Verification items for the finished model (mm, model axes). Face numbers are marked on the shaded views. A direction names the side the tool comes from. Give positions to 0.01 mm unless a question says otherwise; leave off trailing zeros. Loops run counter-clockwise (first coordinate to the right, second up) from the corner with the lowest first, then second, coordinate; pieces in that order, holes last. Notation, with made-up numbers: (-26.75, -14) - (29.25, -14) arc R5 ccw to (29.25, -6) - close; hole circle Ø11 at (-11.5, 60). An arc over 180 degrees is marked (long way). One line per item, written item: value. Start each with the question number.
1. Sectioned sample at B-B (z = -12). Record the cut outline in (x, y), plus the area to 3 significant figures.
2. Sectioned sample at A-A (y = 22). Record the cut outline in (x, z), plus the area to 3 significant figures.
3. Mould release check, pull along Y, two halves, no side actions. Record for the marked faces 4, 5, 6 and 7: pulls with the +Y half, pulls with the -Y half, needs draft (parallel to the pull), parting line crosses it, or undercut.
4. Access from +Z, -Z, +X, -X, +Y, -Y to the whole of each face (thin tool, end or side, straight path). Record for the marked faces 1, 2 and 3.
5. Sectioned sample at D-D (y = 45.5). Record the cut outline in (x, z), plus the area to 3 significant figures.
6. Gauge pin test, flat ends, axial feed: pin 1 (7 mm diameter, centred on y = 31, z = -133.5, fed in from +X); pin 2 (7 mm diameter, centred on y = 31, z = -37.5, fed in from -X); pin 3 (7 mm diameter, centred on x = 31.5, z = -161, fed in from +Y); pin 4 (14 mm diameter, centred on x = 16, y = 51, fed in from +Z). Record the tip position at first contact, or that the pin passes through.
7. Scan lines: L1, parallel to Z at x = 11.5, y = 12.75; L2, parallel to X at y = 9.5, z = -162; L3, parallel to Z at x = 13.5, y = 55. Record each from-to range of solid material in increasing order. Write a range as [from, to].
Autodesk Inventor part; units mm, degrees
ref_plane "Work Plane1" through (23, 0, 0) normal (1, 0, 0) x (0, 1, 0)
ref_plane "Work Plane2" through (0, 0, -87) normal (0, 0, 1) x (1, 0, 0)
ref_plane "XZ Plane" through (0, 0, 0) normal (0, 1, 0) x (-1, 0, 0)
sketch "Sketch1" plane through (0, 0, 0) normal (0, 1, 0) x (-1, 0, 0)
  line L0 (0, 0) -> (-46, 0)
  line L1 (-46, 0) -> (-46, -174)
  line L2 (-46, -174) -> (0, -174)
  line L3 (0, -174) -> (0, 0)
  dimension "d0" = 46
  dimension "d1" = 174
extrude "Extrusion1" add sketch "Sketch1" along normal blind 18
sketch "Sketch2" plane through (0, 18, 0) normal (0, 1, 0) x (1, 0, 0)
  line L0 (0, 0) -> (0, 24)
  line L1 (0, 174) -> (0, 0)
  line L2 (46, 0) -> (46, 174)
  line L3 (0, 24) -> (46, 24)
  line L4 (46, 24) -> (46, 55)
  line L5 (46, 55) -> (0, 55)
  line L6 (0, 55) -> (0, 24)
  line L7 (0, 174) -> (0, 150)
  line L8 (0, 150) -> (46, 150)
  line L9 (46, 150) -> (46, 119)
  line L10 (46, 119) -> (0, 119)
  line L11 (0, 119) -> (0, 150)
  dimension "d4" = 24
  dimension "d5" = 31
  dimension "d6" = 24
  dimension "d7" = 31
extrude "Extrusion2" cut sketch "Sketch2" against normal blind 4 contours L8 L2 L10 L1 | L5 L2 L3 L1
fillet "Fillet1" radius 4 4 edges at (23, 14, -24) (23, 14, -119) (23, 14, -55) (23, 14, -150)
sketch "Sketch3" plane through (0, 18, 0) normal (0, 1, 0) x (1, 0, 0)
  line L0 (46, 150) -> (46, 174)
  line L1 (46, 162) -> (0, 162)
  line L2 (46, 174) -> (0, 174)
  line L3 (23, 174) -> (23, 150)
  line L4 (23, 174) -> (34.5, 174)
  line L5 (34.5, 174) -> (34.5, 150)
  line L6 (0, 150) -> (46, 150)
  line L7 (23, 174) -> (11.5, 174)
  line L8 (11.5, 174) -> (11.5, 150)
  line L9 (0, 0) -> (46, 0)
  line L10 (23, 0) -> (23, 24)
  line L11 (46, 24) -> (0, 24)
  line L12 (46, 0) -> (46, 174)
  line L13 (46, 12) -> (0, 12)
  line L14 (34.5, 0) -> (34.5, 24)
  line L15 (11.5, 0) -> (11.5, 24)
  circle A0 centre (34.5, 12) radius 4
  circle A1 centre (11.5, 12) radius 4
  circle A2 centre (34.5, 162) radius 4
  circle A3 centre (11.5, 162) radius 4
  dimension "d11" = 11.5
  dimension "d12" = 11.5
  dimension "d13" = 8
  dimension "d14" = 8
  dimension "d15" = 8
  dimension "d16" = 8
hole "Hole1" at (34.5, 18, -12) at (11.5, 18, -12) at (34.5, 18, -162) at (11.5, 18, -162) direction (0, -1, 0) diameter 8 depth 18 tip angle 120
sketch "Sketch4" plane through (0, 18, 0) normal (0, 1, 0) x (1, 0, 0)
  line L0 (0, 55) -> (46, 55)
  line L1 (46, 0) -> (46, 174)
  line L2 (0, 55) -> (46, 55)
  line L3 (46, 55) -> (46, 69)
  line L4 (46, 69) -> (0, 69)
  line L5 (0, 69) -> (0, 55)
  line L6 (46, 119) -> (0, 119)
  line L7 (0, 119) -> (46, 119)
  line L8 (46, 119) -> (46, 105)
  line L9 (46, 105) -> (0, 105)
  line L10 (0, 105) -> (0, 119)
  point P0 (0, 0)
  dimension "d24" = 14
  dimension "d25" = 14
extrude "Extrusion3" add sketch "Sketch4" along normal blind 32
sketch "Sketch8" plane through (46, 18, -119) normal (0, 0, -1) x (-1, 0, 0)
  line L0 (0, 32) -> (46, 32)
  circle A0 centre (23, 32) radius 23
  point P0 (46, -18)
  dimension "d35" = 46
sketch "Sketch9" plane through (0, 18, -55) normal (0, 0, 1) x (1, 0, 0)
  line L0 (46, 32) -> (0, 32)
  circle A0 centre (23, 32) radius 23
  point P0 (0, -18)
  dimension "d36" = 46
extrude "Extrusion6" add sketch "Sketch9" against normal blind 14 contours L0 A0 picked at (25.7186, 39.1685)
extrude "Extrusion7" add sketch "Sketch8" against normal blind 14 contours A0 L0 picked at (25.7186, 39.1685)
sketch "Sketch14" plane through (46, 18, -69) normal (0, 0, -1) x (-1, 0, 0)
  line L0 (0, -18) -> (46, -18)
  line L1 (0, -18) -> (0, 32)
  line L2 (0, 32) -> (46, 32)
  circle A0 centre (23, 32) radius 14
  dimension "d51" = 50
  dimension "d52" = 28
extrude "Extrusion10" add sketch "Sketch14" along normal blind 2
sketch "Sketch15" plane through (0, 18, -105) normal (0, 0, 1) x (1, 0, 0)
  line L0 (0, -18) -> (0, 32)
  line L1 (0, 32) -> (46.1632, 32)
  line L2 (0, -18) -> (0, 0)
  circle A0 centre (23.0816, 32) radius 14
  dimension "d55" = 50
  dimension "d56" = 28
extrude "Extrusion11" add sketch "Sketch15" along normal blind 2
sketch "Sketch16" plane through (23, 50, -71) normal (0, 0, -1) x (-1, 0, 0)
  circle A0 centre (0, 0) radius 7
  point P0 (23, -50)
  dimension "d59" = 14
extrude "Extrusion12" cut sketch "Sketch16" against normal blind 16
sketch "Sketch17" plane through (23.0816, 50, -103) normal (0, 0, 1) x (1, 0, 0)
  circle A0 centre (0, 0) radius 7
  point P0 (-23.0816, -50)
  dimension "d62" = 14
extrude "Extrusion13" cut sketch "Sketch17" against normal blind 16
ref_plane "Work Plane1" through (23, 0, 0) normal (1, 0, 0) x (0, 1, 0)
sketch "Sketch21" plane through (23, 0, 0) normal (1, 0, 0) x (0, 1, 0)
  line L0 (18, -55) -> (50, -55)
  line L1 (50, -55) -> (38, -55)
  line L2 (38, -55) -> (14, -55)
  line L3 (14, -55) -> (14, -24)
  arc A0 (18, -24) -> (14, -28) centre (18, -28) ccw
  line L4 (14, -24) -> (18, -24)
  line L5 (18, -24) -> (38, -55)
  line L6 (14, -55) -> (38, -55)
  line L7 (18, -24) -> (14, -24)
  line L8 (14, -55) -> (14, -24)
  line L9 (18, -24) -> (14, -24)
  point P0 (0, 0)
  dimension "d73" = 12
extrude "Extrusion16" add sketch "Sketch21" along normal mid plane 10 contours L2 L3 A0 L5 L0
ref_plane "Work Plane2" through (0, 0, -87) normal (0, 0, 1) x (1, 0, 0)
mirror "Mirror1" about plane through (0, 0, -87) normal (0, 0, 1) of "Extrusion16"
properties part number "Semelle" material "Iron, Cast"
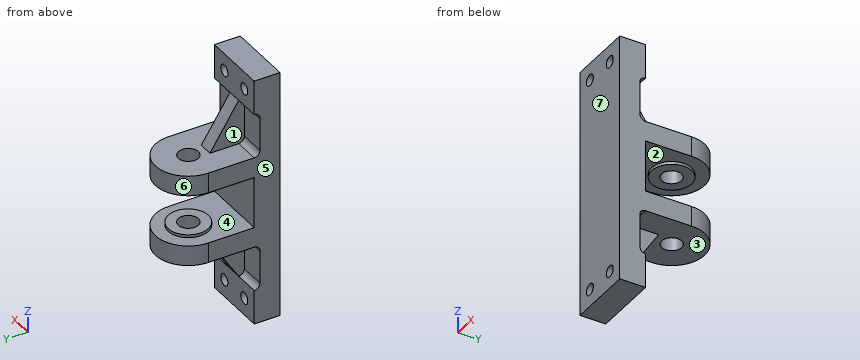
Results are:
1. outline: (0, 0) - (7.5, 0) - (7.5, 18) - (0, 18) - close; (15.5, 0) - (30.5, 0) - (30.5, 18) - (15.5, 18) - close; (38.5, 0) - (46, 0) - (46, 18) - (38.5, 18) - close
1. area: 540 mm^2
2. outline: (0, -119) - (18, -119) - (18, -143.8) - (28, -143.8) - (28, -119) - (46, -119) - (46, -105) - (0, -105) - close; (0, -69) - (46, -69) - (46, -55) - (28, -55) - (28, -30.2) - (18, -30.2) - (18, -55) - (0, -55) - close
2. area: 1,780 mm^2
3. face 4: undercut
3. face 5: needs draft
3. face 6: pulls with the +Y half
3. face 7: pulls with the -Y half
4. face 1: -X, +Y
4. face 2: none
4. face 3: -Z, +Y
5. outline: (0, -119) - (17.72, -119) - (17.72, -103) - (9.82, -103) - (9.82, -105) - (0, -105) - close; (0, -69) - (9.74, -69) - (9.74, -71) - (17.64, -71) - (17.64, -55) - (0, -55) - close; (28.36, -71) - (36.26, -71) - (36.26, -69) - (46, -69) - (46, -55) - (28.36, -55) - close; (28.44, -119) - (46, -119) - (46, -105) - (36.34, -105) - (36.34, -103) - (28.44, -103) - close
5. area: 1,050 mm^2
6. pin 1: stops at x = 28
6. pin 2: passes through
6. pin 3: stops at y = 18
6. pin 4: stops at z = -55
7. L1: z = [-174, -166], [-158, -16], [-8, 0]
7. L2: x = [0, 7.5], [15.5, 30.5], [38.5, 46]
7. L3: z = [-119, -103], [-71, -55]
